Part model, mm, in its own coordinate system. A direction names the side the tool comes from. Round coordinates to 2 decimals unless told otherwise and drop trailing zeros. Write each loop counter-clockwise with the first axis right and the second up, starting at its lowest first coordinate (ties: lowest second). Pieces come first, ordered by that corner, then holes. Notation, with made-up numbers: (-8, -21.5) -> (41, -21.5) arc R24 cw to (41, 2.5) -> close; hole circle Ø9 at (-21.75, -28.75). An arc over 180 degrees is marked (long way). Use CSV: the item, a comma, the result in double quotes. Start each with the question number.
(1) Probe line 1 (X direction, y = 50, z = -3.75); line 2 (Z direction, x = 7, y = 18). List the from-to ranges inside material, lowest first. Write a range as [from, to].
(2) Drop flat-ended pins along their axis: pin 1 (2 mm diameter, centred on x = 40.5, y = -10, fed in from +Z); pin 2 (8 mm diameter, centred on x = 47.5, z = -4.5, fed in from +Y); pin 3 (12 mm diameter, centred on y = -3.5, z = 638.5, fed in from +X). Give the stop position or say it passes through.
(3) Which spindle directions (+Z, -Z, +X, -X, +Y, -Y) get a long thin tool onto all of the face, cutting with end or side? Do faces 5 (the flat face through (25, 0, 769)), 6 (the flat face through (5, 6, 1560)), 7 (the flat face through (0, 0, 0)). Say none if no direction does.
(4) Two-plate mould, pull along Y, no slides. Class faces 1 (the flat face through (-4, -25, 786)), 2 (the flat face through (0, 25, 769)), 3 (the flat face through (-20, 0, 764)), 4 (the flat face through (13, 13, -10)): released by +Y, released by -Y, zero draft, split by the parting line, or undercut.
(5) Saw through at A-A (z = 274). Give the cut face in (x, y), plus the area to 3 significant figures.
```python
from build123d import *

# Parameters (mm, degrees)
F0_W     = 40
F0_H     = 40
F1_DEPTH = 1550
F2_R     = 6.5
F3_DEPTH = 10
F4_R     = 6.5
F5_DEPTH = 10


with BuildPart() as f1:
    # F0 (on Top) → F1 (new body)
    with BuildSketch(Plane.XY):
        with BuildLine():
            Line((-20, -25), (20, -25))
            ThreePointArc((20, -25), (23.535534, -23.535534), (25, -20))
            Line((25, -20), (25, 20))
            ThreePointArc((25, 20), (23.535534, 23.535534), (20, 25))
            Line((20, 25), (-20, 25))
            ThreePointArc((-20, 25), (-23.535534, 23.535534), (-25, 20))
            Line((-25, 20), (-25, -20))
            ThreePointArc((-25, -20), (-23.535534, -23.535534), (-20, -25))
        make_face()
        Rectangle(F0_W, F0_H, mode=Mode.SUBTRACT)
    extrude(amount=F1_DEPTH)

    # F2 (on face) → F3 (join)
    with BuildSketch(Plane.XY.offset(1550)):
        with BuildLine():
            Line((20, 25), (-20, 25))
            ThreePointArc((-20, 25), (-23.535534, 23.535534), (-25, 20))
            Line((-25, 20), (-25, -20))
            ThreePointArc((-25, -20), (-23.535534, -23.535534), (-20, -25))
            Line((-20, -25), (20, -25))
            ThreePointArc((20, -25), (23.535534, -23.535534), (25, -20))
            Line((25, -20), (25, 20))
            ThreePointArc((25, 20), (23.535534, 23.535534), (20, 25))
        make_face()
        Circle(F2_R, mode=Mode.SUBTRACT)
    extrude(amount=F3_DEPTH)

    # F4 (on face) → F5 (join)
    with BuildSketch(Plane(origin=(0, 0, 0), x_dir=(1, 0, 0), z_dir=(0, 0, -1))):
        with BuildLine():
            ThreePointArc((-20, 25), (-23.535534, 23.535534), (-25, 20))
            Line((-25, 20), (-25, -75))
            Line((-25, -75), (25, -75))
            Line((25, -75), (25, -25))
            Line((25, -25), (75, -25))
            Line((75, -25), (75, 25))
            Line((75, 25), (-20, 25))
        make_face()
        with Locations((0, -50)):
            Circle(F4_R, mode=Mode.SUBTRACT)
        with Locations((50, 0)):
            Circle(F4_R, mode=Mode.SUBTRACT)
    extrude(amount=F5_DEPTH)


solid = f1.part
```
Answers:
1,line 1,"x = [-25, -6.5], [6.5, 25]"
1,line 2,"z = [-10, 0], [1550, 1560]"
2,pin 1,"stops at z = 0"
2,pin 2,"stops at y = 25"
2,pin 3,"stops at x = 25"
3,face 5,"+Z, +X, +Y, -Y"
3,face 6,"+Z, +X, -X, +Y, -Y"
3,face 7,"none"
4,face 1,"released by -Y"
4,face 2,"released by +Y"
4,face 3,"undercut"
4,face 4,"zero draft"
5,outline,"(-25, -20) arc R5 ccw to (-20, -25) -> (20, -25) arc R5 ccw to (25, -20) -> (25, 20) arc R5 ccw to (20, 25) -> (-20, 25) arc R5 ccw to (-25, 20) -> close; hole (-20, -20) -> (20, -20) -> (20, 20) -> (-20, 20) -> close"
5,area,"879 mm²"
